```python
from build123d import *

# Parameters (mm, degrees)
PAD_DEPTH       = 12
POCKET_DEPTH    = 10
FILLET_R        = 5
FILLET001_R     = 6
SKETCH002_W     = 211.472893
SKETCH002_H     = 45.806395
POCKET001_DEPTH = 2
SKETCH003_R     = 5
POCKET002_DEPTH = 2.001


with BuildPart() as part:
    # Sketch → Pad (new body)
    with BuildSketch(Plane.XY):
        with BuildLine():
            Line((-90, 12), (89.999964, 12))
            ThreePointArc((90, -12), (102, 1.8e-05), (89.999964, 12))
            Line((-90, -12), (90, -12))
            ThreePointArc((-90, 12), (-102, 0), (-90, -12))
        make_face()
    extrude(amount=PAD_DEPTH)

    # Sketch001 (on Face6 of Pad) → Pocket (cut)
    with BuildSketch(Plane.XY.offset(12)):
        with BuildLine():
            Line((-90, 10), (90, 10))
            ThreePointArc((90, -10), (100, 0), (90, 10))
            Line((-90, -10), (90, -10))
            ThreePointArc((-90, 10), (-100, 0), (-90, -10))
        make_face()
    extrude(amount=-POCKET_DEPTH, mode=Mode.SUBTRACT)

    # Fillet
    fillet_edges = [part.edges().sort_by_distance(p)[0] for p in [
        (0, 10, 2),
    ]]
    fillet(fillet_edges, radius=FILLET_R)

    # Fillet001
    fillet001_edges = [part.edges().sort_by_distance(p)[0] for p in [
        (0, -12, 0),
    ]]
    fillet(fillet001_edges, radius=FILLET001_R)

    # Sketch002 (on Face4 of Fillet001) → Pocket001 (cut)
    with BuildSketch(Plane.XY.offset(12)):
        with Locations((-0.18729, 1.421787)):
            Rectangle(SKETCH002_W, SKETCH002_H)
        with BuildLine():
            Line((-90, 11), (90, 11))
            ThreePointArc((90, -11), (101, 0), (90, 11))
            Line((-90, -11), (90, -11))
            ThreePointArc((-90, 11), (-101, 0), (-90, -11))
        make_face(mode=Mode.SUBTRACT)
    extrude(amount=-POCKET001_DEPTH, mode=Mode.SUBTRACT)

    # Sketch003 (on Face24 of Pocket001) → Pocket002 (cut, through all)
    with BuildSketch(Plane.XY.offset(2)):
        with Locations((-8, 0)):
            Circle(SKETCH003_R)
        with Locations((-24, 0)):
            Circle(SKETCH003_R)
        with Locations((-40, 0)):
            Circle(SKETCH003_R)
        with Locations((-56, 0)):
            Circle(SKETCH003_R)
        with Locations((-72, 0)):
            Circle(SKETCH003_R)
        with Locations((8, 0)):
            Circle(SKETCH003_R)
        with Locations((24, 0)):
            Circle(SKETCH003_R)
        with Locations((40, 0)):
            Circle(SKETCH003_R)
        with Locations((56, 0)):
            Circle(SKETCH003_R)
        with Locations((72, 0)):
            Circle(SKETCH003_R)
    extrude(amount=-POCKET002_DEPTH, mode=Mode.SUBTRACT)


solid = part.part
```
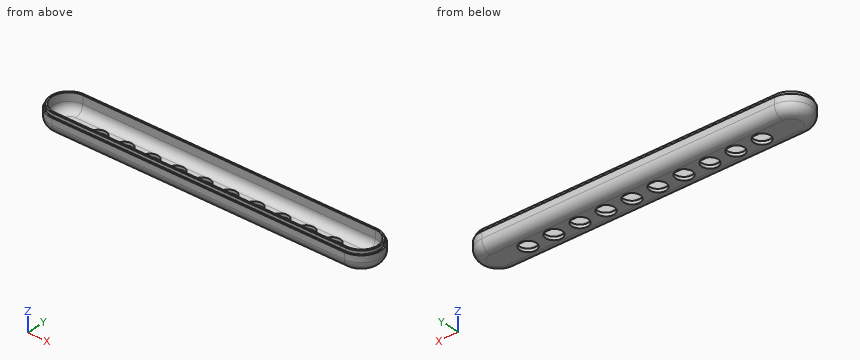
The model under review builds one solid part; all positions refer to its coordinate system, in mm. Coordinates: 2 decimals unless noted, no trailing zeros. Write each loop counter-clockwise with the first axis right and the second up, starting at its lowest first coordinate (ties: lowest second). Pieces come first, ordered by that corner, then holes.
1) To check wall thickness, follow probe 1 along X at (y, z) = (8, 11.5); probe 2 along Y at (x, z) = (72, 1.1); probe 3 along X at (y, z) = (-5.75, 7.75). State the ranges of each line that lie inside material, in increasing order.
2) We need section A-A on x = 69. State the section outline as (y, z) points.
3) We need section B-B on x = -58. State the section outline as (y, z) points.
4) Clearance check with flat-ended pins moving along their axes: pin 1 Ø8 at (x, y) = (-82, 1) entering from +Z; pin 2 Ø11 at (x, y) = (-33, -0.5) entering from +Z; pin 3 Ø11 at (x, y) = (-49, -2.5) entering from +Z; pin 4 Ø3 at (x, z) = (25.5, 4.5) entering from -Y. State where each tip first meets the part, or that it passes through.
Answer list:
1. probe 1: x = -97.55 to -96, 96 to 97.55
1. probe 2: y = -9.46 to -5, 5 to 9.46
1. probe 3: x = -100.53 to -98.18, 98.18 to 100.53
2. outline: (-12, 6) arc R6 ccw to (-6, 0) - (-4, 0) - (-4, 2) - (-5, 2) arc R5 cw to (-10, 7) - (-10, 12) - (-11, 12) - (-11, 10) - (-12, 10) - close; (4, 0) - (6, 0) arc R6 ccw to (12, 6) - (12, 10) - (11, 10) - (11, 12) - (10, 12) - (10, 7) arc R5 cw to (5, 2) - (4, 2) - close
3. outline: (-12, 6) arc R6 ccw to (-6, 0) - (-4.58, 0) - (-4.58, 2) - (-5, 2) arc R5 cw to (-10, 7) - (-10, 12) - (-11, 12) - (-11, 10) - (-12, 10) - close; (4.58, 0) - (6, 0) arc R6 ccw to (12, 6) - (12, 10) - (11, 10) - (11, 12) - (10, 12) - (10, 7) arc R5 cw to (5, 2) - (4.58, 2) - close
4. pin 1: stops at z = 2
4. pin 2: stops at z = 2.1
4. pin 3: stops at z = 3
4. pin 4: stops at y = -12
